```python
from build123d import *

# Parameters (mm, degrees)
F0_R     = 19.05
F1_DEPTH = 6.35
F2_R     = 3.175
F3_DEPTH = 6.35
F4_SIZE  = 0.762
F5_R     = 6.35
F5_R_2   = 2.54
F6_DEPTH = 12.7
F7_SIZE  = 0.381
F8_SIZE  = 6.34999
F9_SIZE  = 2.54


# Not quite as in the source:
# - a fillet or chamfer is up to 0.001 mm smaller than in the source, because OpenCascade refuses the exact size


with BuildPart() as f1:
    # F0 (on Front) → F1 (new body)
    with BuildSketch(Plane.XZ):
        Circle(F0_R)
    extrude(amount=F1_DEPTH)

    # F2 (on face) → F3 (join)
    with BuildSketch(Plane.XZ.offset(6.35)):
        Polygon((-19.05, 25.4), (-25.4, 25.4), (-25.4, -25.4), (25.4, -25.4), (25.4, 25.4), (19.05, 25.4), (19.05, 63.5), (-19.05, 63.5), align=None)
        with Locations((0, 50.8)):
            Circle(F2_R, mode=Mode.SUBTRACT)
    extrude(amount=F3_DEPTH)

    # F4
    f4_edges = [f1.edges().sort_by_distance(p)[0] for p in [
        (-19.05, 0, 0),
    ]]
    chamfer(f4_edges, length=F4_SIZE)

    # F5 (on face) → F6 (cut)
    with BuildSketch(Plane.XZ.offset(12.7)):
        Circle(F5_R)
        with Locations((-19.05, 19.05)):
            Circle(F5_R_2)
        with Locations((19.05, 19.05)):
            Circle(F5_R_2)
        with Locations((19.05, -19.05)):
            Circle(F5_R_2)
        with Locations((-19.05, -19.05)):
            Circle(F5_R_2)
        with Locations((-12.7, 57.15)):
            Circle(F5_R_2)
        with Locations((12.7, 57.15)):
            Circle(F5_R_2)
    extrude(amount=-F6_DEPTH, mode=Mode.SUBTRACT)

    # F7
    f7_edges = [f1.edges().sort_by_distance(p)[0] for p in [
        (-21.59, -12.7, 19.05),
        (16.51, -12.7, 19.05),
        (16.51, -12.7, -19.05),
        (-21.59, -12.7, -19.05),
        (-6.35, -12.7, 0),
        (-6.35, 0, 0),
        (16.51, -6.35, -19.05),
        (-21.59, -6.35, -19.05),
        (-21.59, -6.35, 19.05),
        (16.51, -6.35, 19.05),
        (-15.24, -12.7, 57.15),
        (10.16, -12.7, 57.15),
        (-15.24, -6.35, 57.15),
        (10.16, -6.35, 57.15),
        (-3.175, -6.35, 50.8),
        (-3.175, -12.7, 50.8),
    ]]
    chamfer(f7_edges, length=F7_SIZE)

    # F8 (size 6.35 in the source; OpenCascade refuses exactly that, so slightly less here)
    f8_edges = [f1.edges().sort_by_distance(p)[0] for p in [
        (-19.05, -9.525, 25.4),
        (19.05, -9.525, 25.4),
    ]]
    chamfer(f8_edges, length=F8_SIZE)

    # F9
    f9_edges = [f1.edges().sort_by_distance(p)[0] for p in [
        (-19.05, -9.525, 63.5),
        (19.05, -9.525, 63.5),
    ]]
    chamfer(f9_edges, length=F9_SIZE)


solid = f1.part
```
The model under review builds one solid part; all positions refer to its coordinate system, in mm. A direction names the side the tool comes from. Round coordinates to 2 decimals unless told otherwise and drop trailing zeros. Order: outer loops, then holes, each group sorted by start corner. A loop starts at its lowest first (then second) coordinate and runs counter-clockwise, first axis right, second up.
Item 1: Draft analysis for pull direction X (two halves, no side actions). For faces 3 (the flat face through (-22.2, -9.5, 28.6)), 4 (the flat face through (22.3, -9.5, 28.5)), 5 (the cylindrical face through (-13.25, -9.56, 54.67)), state which applies: released by +X, released by -X, zero draft, split by the parting line, or undercut.
Working result:
face 3: released by -X
face 4: released by +X
face 5: undercut
Item 2: For pin 1 (8 mm diameter, centred on x = -19.05, z = -19.05, fed in from -Y); pin 2 (5 mm diameter, centred on y = -9, z = 46.5, fed in from -X); pin 3 (6.5 mm diameter, centred on x = 12.7, z = 57.15, fed in from +Y); pin 4 (7 mm diameter, centred on y = -8, z = 43.5, fed in from +X), all flat-tipped, find the tip position at first contact; note any pin that passes through.
Working result:
pin 1: stops at y = -12.7
pin 2: stops at x = -19.05
pin 3: stops at y = -6.35
pin 4: stops at x = 19.05
Item 3: Add section D-D, the plane y = -8.5. Count the separate pieces of the cut face and the enclosed holes in it, and give its area (3 significant figures).
Working result:
separate pieces: 1
enclosed holes: 8
area: 3,790 mm2
Item 4: To check wall thickness, follow probe 1 along Z at (x, y) = (0, -10.4) (3 decimals); probe 2 along Z at (x, y) = (0, -3); probe 3 along X at (y, z) = (-7.5, -18.5). State the ranges of each line that lie inside material, in increasing order.
Working result:
probe 1: z = -25.4 to -6.35, 6.35 to 47.625, 53.975 to 63.5
probe 2: z = -19.05 to -6.35, 6.35 to 19.05
probe 3: x = -25.4 to -21.53, -16.57 to 16.57, 21.53 to 25.4
Item 5: Add section A-A, the plane z = 0. State the section outline as (x, y) points.
Working result:
outline: (-25.4, -12.7) - (-6.73, -12.7) - (-6.35, -12.32) - (-6.35, -0.38) - (-6.73, 0) - (-18.29, 0) - (-19.05, -0.76) - (-19.05, -6.35) - (-25.4, -6.35) - close; (6.35, -12.32) - (6.73, -12.7) - (25.4, -12.7) - (25.4, -6.35) - (19.05, -6.35) - (19.05, -0.76) - (18.29, 0) - (6.73, 0) - (6.35, -0.38) - close
Item 6: Add section C-C, the plane z = 57.15. State the section outline as (x, y) points.
Working result:
outline: (-19.05, -12.7) - (-15.62, -12.7) - (-15.24, -12.32) - (-15.24, -6.73) - (-15.62, -6.35) - (-19.05, -6.35) - close; (-10.16, -12.32) - (-9.78, -12.7) - (9.78, -12.7) - (10.16, -12.32) - (10.16, -6.73) - (9.78, -6.35) - (-9.78, -6.35) - (-10.16, -6.73) - close; (15.24, -12.32) - (15.62, -12.7) - (19.05, -12.7) - (19.05, -6.35) - (15.62, -6.35) - (15.24, -6.73) - close
Item 7: Add section B-B, the plane x = 0. State the section outline as (y, z) points (3 decimals), and give its area (3 significant figures).
Working result:
outline: (-12.7, -25.4) - (-6.35, -25.4) - (-6.35, -19.05) - (-0.762, -19.05) - (0, -18.288) - (0, -6.731) - (-0.381, -6.35) - (-12.319, -6.35) - (-12.7, -6.731) - close; (-12.7, 6.731) - (-12.319, 6.35) - (-0.381, 6.35) - (0, 6.731) - (0, 18.288) - (-0.762, 19.05) - (-6.35, 19.05) - (-6.35, 47.244) - (-6.731, 47.625) - (-12.319, 47.625) - (-12.7, 47.244) - close; (-12.7, 54.356) - (-12.319, 53.975) - (-6.731, 53.975) - (-6.35, 54.356) - (-6.35, 63.5) - (-12.7, 63.5) - close
area: 604 mm2
Item 8: Machinability: for faces 1 (the cylindrical face through (12.15, -9.56, 54.67)), 2 (the cylindrical face through (-15.12, -3.52, -11.59)), which of the approach directions +Z, -Z, +X, -X, +Y, -Y give a long, thin tool a straight path to every point of the face, cutting with its end or side? Answer none if there is none.
Working result:
face 1: +Y, -Y
face 2: +Y
